from build123d import *

# Parameters (mm, degrees)
F0_R     = 16.522283
F0_R_2   = 11.25
F1_DEPTH = 3
F2_DEPTH = 10
F3_R     = 2
F4_R     = 2


with BuildPart() as f1:
    # F0 (on Front) → F1 (new body)
    with BuildSketch(Plane.XZ):
        Circle(F0_R)
        Circle(F0_R_2, mode=Mode.SUBTRACT)
    extrude(amount=F1_DEPTH)

    # F0 (on Front) → F2 (join)
    with BuildSketch(Plane.XZ):
        Circle(F0_R_2)
    extrude(amount=F2_DEPTH)

    # F3
    f3_edges = [f1.edges().sort_by_distance(p)[0] for p in [
        (-16.522283, 0, 0),
    ]]
    fillet(f3_edges, radius=F3_R)

    # F4
    f4_edges = [f1.edges().sort_by_distance(p)[0] for p in [
        (-11.25, -10, 0),
    ]]
    fillet(f4_edges, radius=F4_R)


solid = f1.part
Input: part model. Units: mm. Frame: model coordinates. A direction names the side the tool comes from. Coordinates: 2 decimals unless noted, no trailing zeros. Loops run counter-clockwise (first coordinate to the right, second up) from the corner with the lowest first, then second, coordinate; pieces in that order, holes last.
Q1. Contact query for flat-ended pins moving along their axis: pin 1 (4 mm diameter, centred on y = -2.5, z = -6, fed in from -X); pin 2 (5 mm diameter, centred on x = 11, y = -1.5, fed in from +Z); pin 3 (2 mm diameter, centred on x = 9, z = -12.5, fed in from -Y). Output: stop coordinate, or through.
Q2. Cut plane B-B (x = 0). Output: boundary loops of the cut face in (y, z).
Q3. Material intervals for line 1 (Y direction, x = 0, z = -13.5); line 2 (X direction, y = -8.75, z = 1); line 3 (Z direction, x = 0, y = -1.25), sorted ascending.
Q4. Cut plane A-A (z = 0). Output: boundary loops of the cut face in (x, y).
Q5. Cut plane D-D (y = -6). Output: boundary loops of the cut face in (x, z).
Q6. Cut plane C-C (y = -2.5). Output: boundary loops of the cut face in (x, z).
Q7. Set-up query: faces 1 (the face through (0, 0, 0)), 2 (the face through (3, -3, -11)). Return all of +Z, -Z, +X, -X, +Y, -Y with unobstructed straight access to the full face (end or side cutting, diameter ignored); none if empty.
Working result:
1. pin 1: stops at x = -16.03
1. pin 2: stops at z = 14.15
1. pin 3: stops at y = -3
2. outline: (-10, -9.25) arc R2 ccw to (-8, -11.25) - (-3, -11.25) - (-3, -16.52) - (-2, -16.52) arc R2 ccw to (0, -14.52) - (0, 14.52) arc R2 ccw to (-2, 16.52) - (-3, 16.52) - (-3, 11.25) - (-8, 11.25) arc R2 ccw to (-10, 9.25) - close
3. line 1: y = -3 to 0
3. line 2: x = -11.06 to 11.06
3. line 3: z = -16.38 to 16.38
4. outline: (-16.52, -3) - (-11.25, -3) - (-11.25, -8) arc R2 ccw to (-9.25, -10) - (9.25, -10) arc R2 ccw to (11.25, -8) - (11.25, -3) - (16.52, -3) - (16.52, -2) arc R2 ccw to (14.52, 0) - (-14.52, 0) arc R2 ccw to (-16.52, -2) - close
5. outline: circle Ø22.5 at (0, 0)
6. outline: circle Ø33.04 at (0, 0)
7. face 1: +Z, -Z, +X, -X, +Y
7. face 2: -Y
